Build history of the part. All positions in model axes, mm. Round coordinates to 2 decimals unless told otherwise and drop trailing zeros. Write each loop counter-clockwise with the first axis right and the second up, starting at its lowest first coordinate (ties: lowest second). Pieces come first, ordered by that corner, then holes. Notation, with made-up numbers: (73, -0.75) -> (85, -0.75) arc R27 ccw to (85, 15.25) -> close; hole circle Ø5 at (-17, 18.5). An arc over 180 degrees is marked (long way). Return JSON: item names as keys, results as strings.
from build123d import *

# Parameters (mm, degrees)
F0_W     = 78
F0_H     = 223
F1_DEPTH = 1000
F2_SIZE2 = 73
F2_SIZE  = 10
F3_SIZE2 = 73
F3_SIZE  = 45


with BuildPart() as f1:
    # F0 (on Right) → F1 (new body)
    with BuildSketch(Plane.YZ):
        with Locations((-2.6943162084, 52.0490169225)):
            Rectangle(F0_W, F0_H)
    extrude(amount=F1_DEPTH)

    # F2
    f2_edges = [f1.edges().sort_by_distance(p)[0] for p in [
        (500, -41.694316, 163.549017),
    ]]
    f2_side = f1.faces().sort_by_distance((500, -41.694316, 52.049017))[0]
    chamfer(f2_edges, length=F2_SIZE, length2=F2_SIZE2, reference=f2_side)

    # F3
    f3_edges = [f1.edges().sort_by_distance(p)[0] for p in [
        (500, -41.694316, -59.450983),
    ]]
    f3_side = f1.faces().sort_by_distance((500, -2.694316, -59.450983))[0]
    chamfer(f3_edges, length=F3_SIZE, length2=F3_SIZE2, reference=f3_side)


solid = f1.part
Q1. Saw through at C-C on z = 0.5. List the corners of the cut face in (x, y), then the cut area to 3 significant figures.
Verdict:
{"outline": "(0, -33.65) -> (1000, -33.65) -> (1000, 36.31) -> (0, 36.31) -> close", "area": "70,000 mm²"}
Q2. Saw through at B-B on y = -19. List the corners of the cut face in (x, z).
Verdict:
{"outline": "(0, -23.27) -> (1000, -23.27) -> (1000, 156.66) -> (0, 156.66) -> close"}
Q3. Wall check: L1, parallel to Z at x = 882.5, y = 31; L2, parallel to Y at x = 113, z = -21.5; L3, parallel to Z at x = 113, y = -26.5. Give the ranges that are in metal, low to high.
Verdict:
{"L1": "z = -59.45 to 163.51", "L2": "y = -20.09 to 36.31", "L3": "z = -11.1 to 155.63"}
Q4. Pin check, flat tips, straight feed: pin 1 Ø1.5 at (x, z) = (766.5, -28.5) entering from -Y; pin 2 Ø1.5 at (x, y) = (743.5, -17) entering from -Z; pin 3 Ø6 at (x, y) = (434, -25.5) entering from -Z. Stop position of each tip, or through.
Verdict:
{"pin 1": "stops at y = -16.24", "pin 2": "stops at z = -27.73", "pin 3": "stops at z = -17.59"}
Q5. Saw through at A-A on x = 160. List the corners of the cut face in (y, z), then the cut area to 3 significant figures.
Verdict:
{"outline": "(-41.69, 13.55) -> (3.31, -59.45) -> (36.31, -59.45) -> (36.31, 163.55) -> (31.31, 163.55) -> (-41.69, 153.55) -> close", "area": "15,400 mm²"}
